Verification items for the finished model (mm, model axes). A direction names the side the tool comes from. Give positions to 0.01 mm unless a question says otherwise; leave off trailing zeros. Order: outer loops, then holes, each group sorted by start corner. A loop starts at its lowest first (then second) coordinate and runs counter-clockwise, first axis right, second up. Notation, with made-up numbers: (12.5, -37.5) - (32.5, -37.5) arc R10 ccw to (32.5, -20.5) - close; hole circle Ø5 at (41.25, 42.25). An arc over 180 degrees is marked (long way). Answer as a JSON object with one key per item and string values.
Autodesk Inventor part; units mm, degrees
ref_plane "Work Plane1" through (29, 0, 0) normal (0, -1, 0) x (1, 0, 0)
ref_plane "YZ Plane" through (0, 0, 0) normal (1, 0, 0) x (0, 1, 0)
ref_plane "XZ Plane" through (0, 0, 0) normal (0, 1, 0) x (-1, 0, 0)
sketch "Эскиз1" plane through (0, 0, 0) normal (0, 0, 1) x (1, 0, 0)
  line L0 (-1, 0) -> (40, 0)
  line L1 (40, 0) -> (40, 2)
  line L2 (40, 2) -> (26, 2)
  line L3 (26, 2) -> (25.5705, 1.7853)
  line L4 (25.5705, 1.7853) -> (0, 1.7853)
  line L5 (0, 1.7853) -> (0, 3.5)
  line L6 (0, 3.5) -> (-4, 3.5)
  line L7 (-4, 3.5) -> (-4, 1.7321)
  line L8 (-4, 1.7321) -> (-2, 1.7321)
  line L9 (-2, 1.7321) -> (-1, 0)
  line L10 (-12.8, 0) -> (48.8, 0)
  line L11 (0, -0.7) -> (0, 4.2)
  line L12 (26, 2) -> (0, 2) construction
  dimension "d1" = 14
  dimension "d2" = 0.4295
  dimension "d3" = 4
  dimension "d4" = 2
  dimension "d5" = 60
  dimension "d6" = 4
  dimension "d7" = 3.5705
  dimension "d8" = 3.4641
  dimension "d9" = 7
  dimension "d26" = 40
revolve "Базовый элемент" add sketch "Эскиз1" angle 360 about axis through (-1, 0, 0) along (1, 0, 0)
sketch "Эскиз2" plane through (-4, 0, 0) normal (-1, 0, 0) x (0, 0, 1)
  circle A0 centre (0, 0) radius 1.7321
  line L0 (0, -4.9) -> (0, 4.9)
  line L1 (-4.9, 0) -> (4.9, 0)
  line L2 (1.7321, 0) -> (0.866, -1.5)
  line L3 (0.866, -1.5) -> (-0.866, -1.5)
  line L4 (-0.866, -1.5) -> (-1.7321, 0)
  line L5 (-1.7321, 0) -> (-0.866, 1.5)
  line L6 (-0.866, 1.5) -> (0.866, 1.5)
  line L7 (0.866, 1.5) -> (1.7321, 0)
extrude "Паз" add sketch "Эскиз2" against normal up to next contours L7 A0 | A0 L2 | L6 L0 A0 | A0 L0 L3 | L0 L6 A0 | A0 L3 L0 | L4 A0 | A0 L5
fillet "Сопряжение1" radius 0.4 1 edges at (-4, -3.5, 0)
thread "Резьба"
chamfer "Фаска1" distance 0.4294 distance2 0.4294 1 edges at (40, -2, 0) measured on face at (40, -0.1312, -0.9006)
ref_plane "Work Plane1" through (29, 0, 0) normal (0, -1, 0) x (1, 0, 0)
fillet "Fillet2" radius 0.1 1 edges at (0, -1.7853, 0)
equation "\"d1\" = GEL"
equation "\"d3\" = KOH"
equation "\"d4\" = INTI"
equation "\"d6\" = GD"
equation "\"d7\" = BDM"
equation "\"d8\" = 1.1547 * SW"
equation "\"d9\" = KOD"
equation "\"d26\" = NLG"
equation "\"d30\" = R"
equation "\"d17\" = RR"
equation "\"d13\" = GEL"
equation "\"d15\" = -0.5 * SPD + 0.5 * GD"
equation "\"d16\" = GUL"
equation "\"GD\" = NND"
equation "\"NLG\" = 40"
equation "\"GEL\" = 14"
equation "\"KOD\" = 7"
equation "\"KOH\" = NND"
equation "\"INTI\" = 2"
equation "\"GAL\" = 0.61345 * PTC"
equation "\"GUL\" = 0.61345 * PTC"
equation "\"BDM\" = 3.5705"
equation "\"SW\" = 3"
equation "\"RR\" = 0.4"
equation "\"SPD\" = NND - 1.2269 * PTC"
equation "\"R\" = 0.1"
equation "\"PHH\" = 0.4"
equation "\"GD1\" = THREADDIA - 1.2269 * PTC"
equation "\"THREADDIA\" = 4"
equation "\"FAWI\" = 45deg"
equation "\"PTC\" = 0.7"
equation "\"NND\" = 4"
equation "\"TOA\" = 30deg"
equation "\"E0\" = 1.155 * SW"
properties part number "CSN 02 1143 - M4 x 40" material "Сталь, мягкая"
(1) Gauge pin test, flat ends, axial feed: pin 1 Ø2 at (x, y) = (10, 2) entering from -Z; pin 2 Ø4 at (x, y) = (26.5, 2) entering from +Z. Record the tip position at first contact, or that the pin passes through.
Computed values:
{"pin 1": "stops at z = -1.48", "pin 2": "stops at z = 2"}
(2) Release check for a two-part mould opening along X. For faces 1 (the cylindrical face through (12.657, -0.387, 1.743)), 2 (the conical face through (-1, 0, 0)), 3 (the flat face through (-2.948, 0.761, 1.293)) record: pulls with the +X half, pulls with the -X half, needs draft (parallel to the pull), parting line crosses it, or undercut.
Computed values:
{"face 1": "undercut", "face 2": "pulls with the -X half", "face 3": "needs draft"}
(3) Access from +Z, -Z, +X, -X, +Y, -Y to the whole of each face (thin tool, end or side, straight path). Record for faces 4 (the cylindrical face through (-1.825, 3.233, 1.341)), 5 (the cylindrical face through (33, 0, 2)), 6 (the flat face through (-3, -1.5, 0)).
Computed values:
{"face 4": "+X, -X", "face 5": "+X", "face 6": "-X"}
(4) Material ranges on line 1 along X through (y, z) = (-2.25, -0.5); line 2 along Y through (x, z) = (30, 1.25); line 3 along Z through (x, y) = (30, -1), recorded low to high. Write a range as [from, to].
Computed values:
{"line 1": "x = [-4, 0]", "line 2": "y = [-1.56, 1.56]", "line 3": "z = [-1.73, 1.73]"}
(5) Section check A-A (x = 10). Record the cut outline in (y, z), then the cut area to 3 significant figures.
Computed values:
{"outline": "circle Ø3.57 at (0, 0)", "area": "10.0 mm²"}
